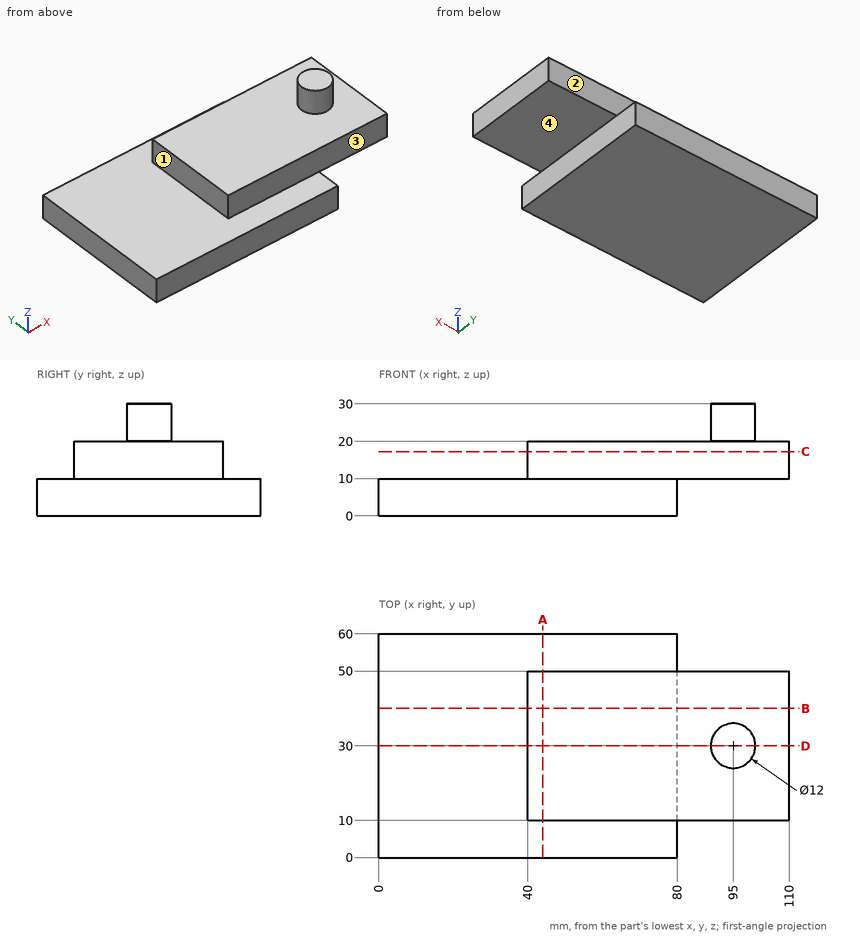
For this review, use the dimensioned drawing (mm, ordinates from the lowest corner) and the shaded views. A direction names the side the tool comes from. Coordinates: 2 decimals unless noted, no trailing zeros. Loops run counter-clockwise (first coordinate to the right, second up) from the corner with the lowest first, then second, coordinate; pieces in that order, holes last.
1. For the marked faces 1, 2, 3 and 4, list the 3-axis set-ups (+Z, -Z, +X, -X, +Y, -Y) from which the entire face can be reached by the end or side of a thin tool; tool diameter is ignored.
2. For line 1 (Z direction, x = 38, y = 48); line 2 (Z direction, x = 71, y = 15.5); line 3 (X direction, y = 34.5, z = 7), list the stretches that pass through material, from the lowest coordinate up.
3. Add section C-C, the plane z = 17.25. Give the boundary of the cut face in (x, y).
4. Insertion check: P1, Ø3, axis at y = 32, z = 4.5, coming from the +X side; P2, Ø6, axis at x = 16, y = 21, coming from the +Z side; P3, Ø6, axis at x = 90.5, z = 27, coming from the +Y side. Each pin has a flat end and moves straight along its axis. Give the tip position at first contact, or say it passes through.
5. Add section B-B, the plane y = 40. Give the boundary of the cut face in (x, z).
6. Add section D-D, the plane y = 30. Give the boundary of the cut face in (x, z), then the cut area to 3 significant figures.
7. Add section A-A, the plane x = 44. Give the boundary of the cut face in (y, z), then the cut area to 3 significant figures.
Result:
1. face 1: +Z, -X, +Y, -Y
1. face 2: +Z, +X, -X, +Y
1. face 3: +Z, +X, -X, -Y
1. face 4: -Z, +X, +Y, -Y
2. line 1: z = 0 to 10
2. line 2: z = 0 to 20
2. line 3: x = 0 to 80
3. outline: (40, 10) - (110, 10) - (110, 50) - (40, 50) - close
4. P1: stops at x = 80
4. P2: stops at z = 10
4. P3: stops at y = 35.81
5. outline: (0, 0) - (80, 0) - (80, 10) - (110, 10) - (110, 20) - (40, 20) - (40, 10) - (0, 10) - close
6. outline: (0, 0) - (80, 0) - (80, 10) - (110, 10) - (110, 20) - (101, 20) - (101, 30) - (89, 30) - (89, 20) - (40, 20) - (40, 10) - (0, 10) - close
6. area: 1,620 mm2
7. outline: (0, 0) - (60, 0) - (60, 10) - (50, 10) - (50, 20) - (10, 20) - (10, 10) - (0, 10) - close
7. area: 1,000 mm2
